Geometry check sheet. Reference: drawing and pictorial views, mm from the part's lowest x, y, z. A direction names the side the tool comes from. Coordinates: 2 decimals unless noted, no trailing zeros. Order: outer loops, then holes, each group sorted by start corner. A loop starts at its lowest first (then second) coordinate and runs counter-clockwise, first axis right, second up. Notation, with made-up numbers: M 14.25,-17.75 L 39.25,-17.75 A7 ccw 39.25,-9.75 Z; hole C 72.25,23.25 d10. An arc over 180 degrees is marked long. Return JSON: item names as keys, results as strings.
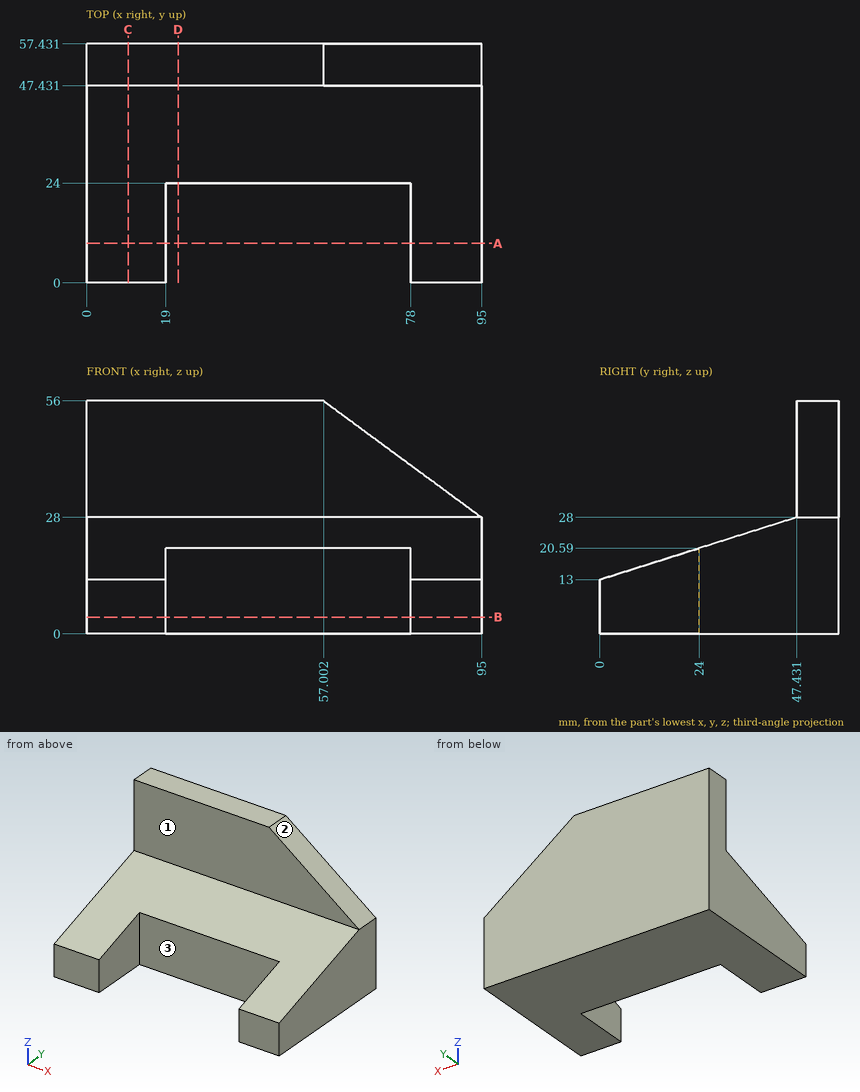
Q1. Cross-section at C-C, the plane x = 10. Record the boundary of the cut face in (y, z), and give its area (3 significant figures).
Values:
{"outline": "M 0,0 L 57.43,0 L 57.43,56 L 47.43,56 L 47.43,28 L 0,13 Z", "area": "1,530 mm^2"}
Q2. Tool access check on the marked faces 1, 2 and 3. Record the directions out of +Z, -Z, +X, -X, +Y, -Y that give a thin tool (end or side, any length) a straight path to the whole face; none if there is none.
Values:
{"face 1": "+Z, +X, -X, -Y", "face 2": "+Z, +X, +Y, -Y", "face 3": "+Z, -Z, -Y"}
Q3. Cross-section at B-B, the plane z = 4. Record the boundary of the cut face in (x, y).
Values:
{"outline": "M 0,0 L 19,0 L 19,24 L 78,24 L 78,0 L 95,0 L 95,57.43 L 0,57.43 Z"}
Q4. Go/stop test with flat-tipped pins: pin 1 (6 mm diameter, centred on x = 35, y = 34.5, fed in from +Z); pin 2 (1.5 mm diameter, centred on x = 23, z = 49.5, fed in from -Y); pin 3 (1.5 mm diameter, centred on x = 80.5, z = 40, fed in from -Y); pin 4 (6 mm diameter, centred on x = 48.5, z = 7.5, fed in from -Y). Record where each tip stops, or that it passes through.
Values:
{"pin 1": "z = 24.86", "pin 2": "y = 47.43", "pin 3": "through", "pin 4": "y = 24"}
Q5. Material ranges on line 1 along X through (y, z) = (13, 13.5); line 2 along Y through (x, z) = (64, 40); line 3 along Z through (x, y) = (60, 51), recorded low to high.
Values:
{"line 1": "0 to 19, 78 to 95", "line 2": "47.43 to 57.43", "line 3": "0 to 53.79"}
Q6. Cross-section at A-A, the plane y = 9.5. Record the boundary of the cut face in (x, z) (1 decimal), and give its area (3 significant figures).
Values:
{"outline": "M 0,0 L 19,0 L 19,16 L 0,16 Z; M 78,0 L 95,0 L 95,16 L 78,16 Z", "area": "576 mm^2"}
Q7. Cross-section at D-D, the plane x = 22. Record the boundary of the cut face in (y, z), and give its area (3 significant figures).
Values:
{"outline": "M 24,0 L 57.43,0 L 57.43,56 L 47.43,56 L 47.43,28 L 24,20.59 Z", "area": "1,130 mm^2"}
